```python
from build123d import *

# Parameters (mm, degrees)
BOSS_EXTRUDE1_DEPTH = 40
CUT_EXTRUDE1_REACH  = 27
SKETCH2_R           = 2.25
CUT_EXTRUDE2_REACH  = 7
SKETCH3_R           = 2.25
SKETCH4_R           = 3.75
CUT_EXTRUDE3_DEPTH  = 2
SKETCH5_R           = 3.75
CUT_EXTRUDE4_DEPTH  = 2
CHAMFER1_SIZE       = 3


with BuildPart() as part:
    # Sketch1 → Boss-Extrude1 (new body)
    with BuildSketch(Plane(origin=(0, 0, 0), x_dir=(1, 0, 0), z_dir=(0, 1, 0))):
        Polygon((0, 0), (25, 0), (25, 5), (5, 5), (5, 20), (0, 20), align=None)
    extrude(amount=BOSS_EXTRUDE1_DEPTH)

    # Sketch2 → Cut-Extrude1 (cut, up to next)
    with BuildSketch(Plane.ZY, mode=Mode.PRIVATE) as cut_extrude1_sk1:
        with Locations((-10, 10)):
            Circle(SKETCH2_R)
    cut_extrude1_tool1 = extrude(cut_extrude1_sk1.sketch, amount=-CUT_EXTRUDE1_REACH, mode=Mode.PRIVATE) & part.part
    add(cut_extrude1_tool1.solids().sort_by_distance((0, 10, -10))[0], mode=Mode.SUBTRACT)
    # Sketch2 → Cut-Extrude1 (cut, up to next)
    with BuildSketch(Plane.ZY, mode=Mode.PRIVATE) as cut_extrude1_sk2:
        with Locations((-10, 30)):
            Circle(SKETCH2_R)
    cut_extrude1_tool2 = extrude(cut_extrude1_sk2.sketch, amount=-CUT_EXTRUDE1_REACH, mode=Mode.PRIVATE) & part.part
    add(cut_extrude1_tool2.solids().sort_by_distance((0, 30, -10))[0], mode=Mode.SUBTRACT)

    # Sketch3 → Cut-Extrude2 (cut, up to next)
    with BuildSketch(Plane(origin=(0, 0, -5), x_dir=(-1, 0, 0), z_dir=(0, 0, -1)), mode=Mode.PRIVATE) as cut_extrude2_sk1:
        with Locations((-15, 10)):
            Circle(SKETCH3_R)
    cut_extrude2_tool1 = extrude(cut_extrude2_sk1.sketch, amount=-CUT_EXTRUDE2_REACH, mode=Mode.PRIVATE) & part.part
    add(cut_extrude2_tool1.solids().sort_by_distance((15, 10, -5))[0], mode=Mode.SUBTRACT)
    # Sketch3 → Cut-Extrude2 (cut, up to next)
    with BuildSketch(Plane(origin=(0, 0, -5), x_dir=(-1, 0, 0), z_dir=(0, 0, -1)), mode=Mode.PRIVATE) as cut_extrude2_sk2:
        with Locations((-15, 30)):
            Circle(SKETCH3_R)
    cut_extrude2_tool2 = extrude(cut_extrude2_sk2.sketch, amount=-CUT_EXTRUDE2_REACH, mode=Mode.PRIVATE) & part.part
    add(cut_extrude2_tool2.solids().sort_by_distance((15, 30, -5))[0], mode=Mode.SUBTRACT)

    # Sketch4 → Cut-Extrude3 (cut)
    with BuildSketch(Plane(origin=(0, 0, -5), x_dir=(-1, 0, 0), z_dir=(0, 0, -1))):
        with Locations((-15, 10)):
            Circle(SKETCH4_R)
        with Locations((-15, 30)):
            Circle(SKETCH4_R)
    extrude(amount=-CUT_EXTRUDE3_DEPTH, mode=Mode.SUBTRACT)

    # Sketch5 → Cut-Extrude4 (cut)
    with BuildSketch(Plane(origin=(5, 0, 0), x_dir=(0, 0, -1), z_dir=(1, 0, 0))):
        with Locations((10, 30)):
            Circle(SKETCH5_R)
        with Locations((10, 10)):
            Circle(SKETCH5_R)
    extrude(amount=-CUT_EXTRUDE4_DEPTH, mode=Mode.SUBTRACT)

    # Chamfer1
    chamfer1_edges = [part.edges().sort_by_distance(p)[0] for p in [
        (25, 40, -2.5),
        (2.5, 40, -20),
        (2.5, 0, -20),
        (25, 0, -2.5),
    ]]
    chamfer(chamfer1_edges, length=CHAMFER1_SIZE)


solid = part.part
```
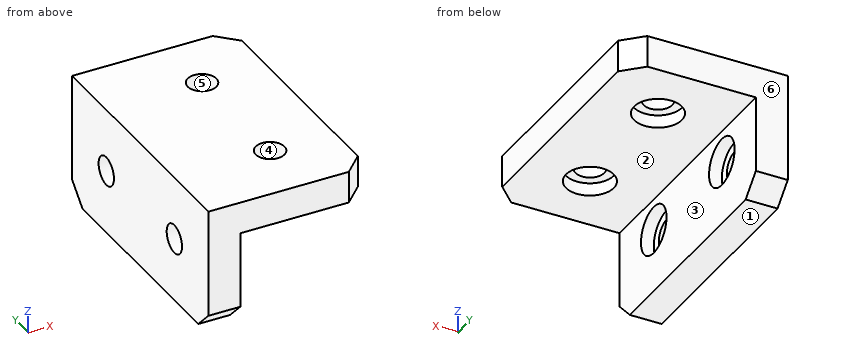
Read the model definition and answer for the solid it produces. Units are mm, in the model's axes. Face numbers are marked on the shaded views. A direction names the side the tool comes from. Round coordinates to 2 decimals unless told otherwise and drop trailing zeros. Write each loop counter-clockwise with the first axis right and the second up, starting at its lowest first coordinate (ties: lowest second). Pieces come first, ordered by that corner, then holes. Notation, with made-up numbers: (22.25, 74) - (36.25, 74) arc R26 cw to (36.25, 99) - close; hole circle Ø1 at (71.5, 15). An arc over 180 degrees is marked (long way). One line per item, written item: value.
Q1. Which of the six approach directions +Z, -Z, +X, -X, +Y, -Y give full straight-line access (tool end or side, diameter ignored) to the marked faces 1 and 2?
The answers:
face 1: -Z, +X, -X, +Y, -Y
face 2: -Z, +X, +Y, -Y
Q2. Find section C-C (y = 30). Determine the outline of the cut face in (x, z), and give its area (3 significant figures).
The answers:
outline: (0, -20) - (5, -20) - (5, -13.75) - (3, -13.75) - (3, -12.25) - (0, -12.25) - close; (0, -7.75) - (3, -7.75) - (3, -6.25) - (5, -6.25) - (5, -5) - (11.25, -5) - (11.25, -3) - (12.75, -3) - (12.75, 0) - (0, 0) - close; (17.25, -3) - (18.75, -3) - (18.75, -5) - (25, -5) - (25, 0) - (17.25, 0) - close
area: 143 mm2
Q3. Find section A-A (z = -10). Determine the outline of the cut face in (x, y).
The answers:
outline: (0, 0) - (5, 0) - (5, 6.25) - (3, 6.25) - (3, 7.75) - (0, 7.75) - close; (0, 12.25) - (3, 12.25) - (3, 13.75) - (5, 13.75) - (5, 26.25) - (3, 26.25) - (3, 27.75) - (0, 27.75) - close; (0, 32.25) - (3, 32.25) - (3, 33.75) - (5, 33.75) - (5, 40) - (0, 40) - close
Q4. Each of these flat-tipped pins is pushed along its axis until it touches: P1, Ø8.5, axis at y = 30, z = -10, coming from the +X side; P2, Ø7, axis at y = 10, z = -10, coming from the +X side; P3, Ø8, axis at x = 15, y = 12, coming from the -Z side. Where does it stop, or does it pass through?
The answers:
P1: stops at x = 5
P2: stops at x = 3
P3: stops at z = -5
Q5. For a pull along X with two mould halves and no side action, classify the marked faces 3, 4, 5 and 6 as pulls with the +X half, pulls with the -X half, needs draft (parallel to the pull), parting line crosses it, or undercut.
The answers:
face 3: pulls with the +X half
face 4: undercut
face 5: undercut
face 6: needs draft
Q6. Find section B-B (x = 15). Determine the outline of the cut face in (y, z), and give its area (3 significant figures).
The answers:
outline: (0, -5) - (6.25, -5) - (6.25, -3) - (7.75, -3) - (7.75, 0) - (0, 0) - close; (12.25, -3) - (13.75, -3) - (13.75, -5) - (26.25, -5) - (26.25, -3) - (27.75, -3) - (27.75, 0) - (12.25, 0) - close; (32.25, -3) - (33.75, -3) - (33.75, -5) - (40, -5) - (40, 0) - (32.25, 0) - close
area: 143 mm2
Q7. Find section D-D (y = 3.5). Determine the outline of the cut face in (x, z), and give its area (3 significant figures).
The answers:
outline: (0, -20) - (5, -20) - (5, -5) - (25, -5) - (25, 0) - (0, 0) - close
area: 200 mm2
Q8. Straight lines are drawn through the part: line 1 (Y direction, x = 4.2, z = -10); line 2 (X direction, y = 20.5, z = -5.5); line 3 (Z direction, x = 19.5, y = 23.5). For each, find the intervals that lie inside material, in ascending order. Write a range as from..to.
The answers:
line 1: y = 0..6.25, 13.75..26.25, 33.75..40
line 2: x = 0..5
line 3: z = -5..0
